Verification items for the finished model (mm, model axes). A direction names the side the tool comes from. Coordinates: 2 decimals unless noted, no trailing zeros. Write each loop counter-clockwise with the first axis right and the second up, starting at its lowest first coordinate (ties: lowest second). Pieces come first, ordered by that corner, then holes. Notation, with made-up numbers: (52, 88.5) -> (89, 88.5) arc R35 ccw to (89, 120.5) -> close; hole circle Ø6 at (-19.75, 75.5). An arc over 180 degrees is marked (long way). Answer in a Markdown table with one row per item.
```python
from build123d import *

# Parameters (mm, degrees)
F0_W     = 260
F0_H     = 430
F1_DEPTH = 130
F2_W     = 256
F2_H     = 426
F3_DEPTH = 129
F4_R     = 2


with BuildPart() as f1:
    # F0 (on Front) → F1 (new body)
    with BuildSketch(Plane.XZ):
        Rectangle(F0_W, F0_H)
    extrude(amount=F1_DEPTH)

    # F2 (on face) → F3 (cut)
    with BuildSketch(Plane.XZ.offset(130)):
        Rectangle(F2_W, F2_H)
    extrude(amount=-F3_DEPTH, mode=Mode.SUBTRACT)

    # F4
    f4_edges = [f1.edges().sort_by_distance(p)[0] for p in [
        (-130, -65, 215),
        (130, -65, 215),
        (-130, -65, -215),
        (130, -65, -215),
        (0, 0, -215),
        (130, 0, 0),
        (-130, 0, 0),
        (0, 0, 215),
    ]]
    fillet(f4_edges, radius=F4_R)


solid = f1.part
```
1. Mould release check, pull along X, two halves, no side actions. Record for faces 1 (the flat face through (-2, -1, 3)), 2 (the flat face through (-2, 0, 3)), 3 (the flat face through (-130, -65, -3)): released by +X, released by -X, zero draft, split by the parting line, or undercut.
Geometry says:
| item | result |
|---|---|
| face 1 | undercut |
| face 2 | zero draft |
| face 3 | released by -X |
2. Section check B-B, the plane y = -55. Record the boundary of the cut face in (x, z), plus the area to 3 significant figures.
Geometry says:
| item | result |
|---|---|
| outline | (-130, -213) arc R2 ccw to (-128, -215) -> (128, -215) arc R2 ccw to (130, -213) -> (130, 213) arc R2 ccw to (128, 215) -> (-128, 215) arc R2 ccw to (-130, 213) -> close; hole (-128, -213) -> (128, -213) -> (128, 213) -> (-128, 213) -> close |
| area | 2,740 mm^2 |
3. Section check A-A, the plane x = -109.5. Record the boundary of the cut face in (y, z).
Geometry says:
| item | result |
|---|---|
| outline | (-130, -215) -> (-2, -215) arc R2 ccw to (0, -213) -> (0, 213) arc R2 ccw to (-2, 215) -> (-130, 215) -> (-130, 213) -> (-1, 213) -> (-1, -213) -> (-130, -213) -> close |
4. Section check C-C, the plane z = 24. Record the boundary of the cut face in (x, y), plus the area to 3 significant figures.
Geometry says:
| item | result |
|---|---|
| outline | (-130, -130) -> (-128, -130) -> (-128, -1) -> (128, -1) -> (128, -130) -> (130, -130) -> (130, -2) arc R2 ccw to (128, 0) -> (-128, 0) arc R2 ccw to (-130, -2) -> close |
| area | 774 mm^2 |
5. Tool access check on faces 4 (the flat face through (-2, -65, -215)), 5 (the flat face through (128, -66, -3)). Record the directions out of +Z, -Z, +X, -X, +Y, -Y that give a thin tool (end or side, any length) a straight path to the whole face; none if there is none.
Geometry says:
| item | result |
|---|---|
| face 4 | -Z, +X, -X, +Y, -Y |
| face 5 | -Y |
6. Thickness scan on line 1 (X direction, y = -85.5, z = 192.5); line 2 (Z direction, x = -94.5, y = -122); line 3 (Y direction, x = -52, z = 65). Record the ranges inside material, lowest first. Write a range as from..to.
Geometry says:
| item | result |
|---|---|
| line 1 | -130..-128, 128..130 |
| line 2 | -215..-213, 213..215 |
| line 3 | -1..0 |
7. Depth check by flat-ended pin: P1, Ø2, axis at x = 103, z = 24, coming from the -Y side. Enter the tip coordinate at first touch or a pass-through.
Geometry says:
| item | result |
|---|---|
| P1 | y = -1 |
